Geometry check sheet. Reference: drawing and pictorial views, mm from the part's lowest x, y, z. Coordinates: 2 decimals unless noted, no trailing zeros. Write each loop counter-clockwise with the first axis right and the second up, starting at its lowest first coordinate (ties: lowest second). Pieces come first, ordered by that corner, then holes. Notation, with made-up numbers: M -37,57.25 L -7,57.25 A28 cw -7,95.25 Z; hole C 83.5,83.5 d11. An arc over 180 degrees is marked long. One line per item, written item: value.
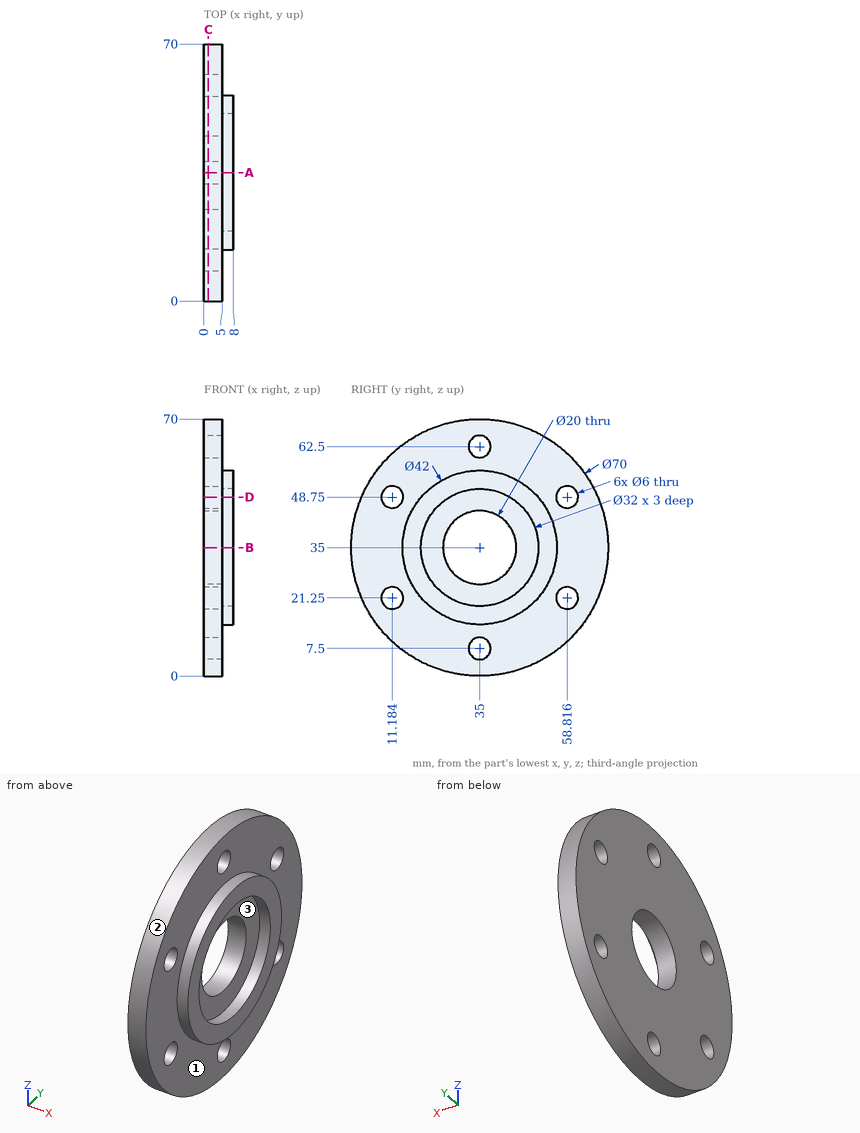
Item 1: Cross-section at C-C, the plane x = 1.25. Enter the section's corners in (y, z).
The answers:
outline: C 35,35 d70; hole C 11.18,21.25 d6; hole C 11.18,48.75 d6; hole C 35,35 d20; hole C 35,7.5 d6; hole C 35,62.5 d6; hole C 58.82,21.25 d6; hole C 58.82,48.75 d6
Item 2: Scan lines: line 1 (Z direction, x = 3, y = 10) (1 decimal); line 2 (Y direction, x = 1.95, z = 48.75) (1 decimal); line 3 (X direction, y = 30, z = 12.5). Record each from-to range of solid material in increasing order.
The answers:
line 1: z = 10.5 to 18.5, 24 to 46, 51.5 to 59.5
line 2: y = 2.8 to 8.2, 14.2 to 55.8, 61.8 to 67.2
line 3: x = 0 to 5
Item 3: Draft check along Z on the marked faces 1, 2 and 3. Enter one of: released by +Z, released by -Z, zero draft, split by the parting line, or undercut.
The answers:
face 1: zero draft
face 2: split by the parting line
face 3: undercut
Item 4: Cross-section at B-B, the plane z = 35. Enter the section's corners in (x, y).
The answers:
outline: M 0,0 L 5,0 L 5,14 L 8,14 L 8,19 L 5,19 L 5,25 L 0,25 Z; M 0,45 L 5,45 L 5,51 L 8,51 L 8,56 L 5,56 L 5,70 L 0,70 Z
Item 5: Go/stop test with flat-tipped pins: P1, Ø2, axis at x = 3, z = 26, coming from the -Y side; P2, Ø5, axis at y = 58.82, z = 48.75, coming from the -X side; P3, Ø1.5, axis at x = 6.5, y = 34, coming from the +Z side; P4, Ø3, axis at x = 4.5, y = 61.5, coming from the -Z side (1 decimal). Record where each tip stops, or that it passes through.
The answers:
P1: stops at y = 0.93
P2: passes through
P3: stops at z = 56
P4: stops at z = 10.5
Item 6: Cross-section at D-D, the plane z = 48.75. Enter the section's corners in (x, y), and give its area (3 significant figures).
The answers:
outline: M 0,2.81 L 5,2.81 L 5,8.18 L 0,8.18 Z; M 0,14.18 L 5,14.18 L 5,19.13 L 8,19.13 L 8,26.82 L 5,26.82 L 5,43.18 L 8,43.18 L 8,50.87 L 5,50.87 L 5,55.82 L 0,55.82 Z; M 0,61.82 L 5,61.82 L 5,67.19 L 0,67.19 Z
area: 308 mm²
Item 7: Cross-section at A-A, the plane y = 35. Enter the section's corners in (x, z), and give its area (3 significant figures).
The answers:
outline: M 0,0 L 5,0 L 5,4.5 L 0,4.5 Z; M 0,10.5 L 5,10.5 L 5,14 L 8,14 L 8,19 L 5,19 L 5,25 L 0,25 Z; M 0,45 L 5,45 L 5,51 L 8,51 L 8,56 L 5,56 L 5,59.5 L 0,59.5 Z; M 0,65.5 L 5,65.5 L 5,70 L 0,70 Z
area: 220 mm²
